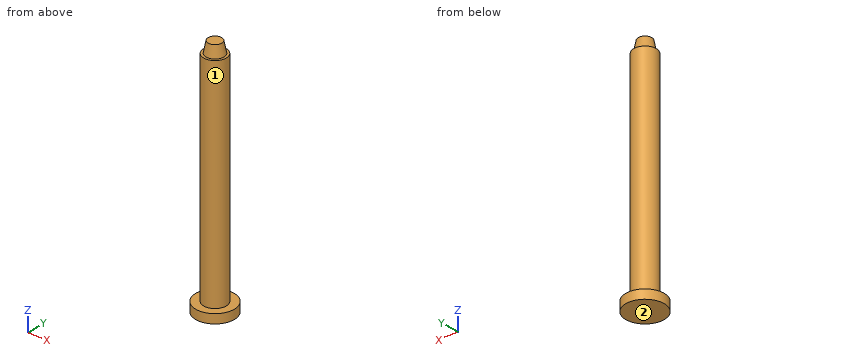
```python
from build123d import *

# Parameters (mm, degrees)
F0_R     = 8.5
F1_DEPTH = 4
F2_R     = 5
F3_DEPTH = 100


with BuildPart() as f1:
    # F0 (on Top) → F1 (new body)
    with BuildSketch(Plane.XY):
        Circle(F0_R)
    extrude(amount=F1_DEPTH)

    # F2 (on Top) → F3 (join)
    with BuildSketch(Plane.XY):
        Circle(F2_R)
    extrude(amount=F3_DEPTH)

    # F4 (on Right) → F5 (revolve)
    with BuildSketch(Plane.YZ):
        Polygon((3, 105), (0, 105), (0, 100), (4, 100), align=None)
    revolve(axis=Axis((0, 0, 102.5), (0, 0, -1)))


solid = f1.part
```
CAD build for the part. Positions are in the model's coordinates, mm. Face numbers are marked on the shaded views. A direction names the side the tool comes from. Coordinates: 2 decimals unless noted, no trailing zeros. Order: outer loops, then holes, each group sorted by start corner. A loop starts at its lowest first (then second) coordinate and runs counter-clockwise, first axis right, second up. Notation, with made-up numbers: M 31,89 L 59,89 A16 ccw 59,108 Z; hole C -1.75,-5 d4. An arc over 180 degrees is marked long. Write each question's results on one line, items separated by ' | '. Start each with the question number.
Q1. Cut at D-D (y = 7). List the corners of the cut face in (x, z).
Q2. Flat gauge pins, fed straight in: P1, Ø5, axis at x = -1, z = 48, coming from the -Y side; P2, Ø4, axis at x = 0.5, z = 82.5, coming from the +Y side; P3, Ø5, axis at x = 6, z = 41, coming from the +Y side. Where does each tip first touch, or does it go through?
Q3. Cut at A-A (x = 0). List the corners of the cut face in (y, z), then the cut area to 3 significant figures.
Q4. Cut at C-C (z = 16.5). List the corners of the cut face in (x, y), then the cut area to 3 significant figures.
Q5. Drill centre lines: probe 1 along Z at (x, y) = (-3.5, -4.75); probe 2 along Y at (x, z) = (4, 65.5); probe 3 along Z at (x, y) = (-4, -2.75). Where is each one in solid material? Low to high. Write a range as from..to.
Q6. Which spindle directions (+Z, -Z, +X, -X, +Y, -Y) get a long thin tool onto all of the face, cutting with end or side? Do the marked faces 1 and 2. Say none if no direction does.
Found:
1) outline: M -4.82,0 L 4.82,0 L 4.82,4 L -4.82,4 Z
2) P1: y = -5 | P2: y = 5 | P3: y = 3.57
3) outline: M -8.5,0 L 8.5,0 L 8.5,4 L 5,4 L 5,100 L 4,100 L 3,105 L -3,105 L -4,100 L -5,100 L -5,4 L -8.5,4 Z | area: 1,060 mm²
4) outline: C 0,0 d10 | area: 78.5 mm²
5) probe 1: 0..4 | probe 2: -3..3 | probe 3: 0..100
6) face 1: +Z | face 2: -Z, +X, -X, +Y, -Y
